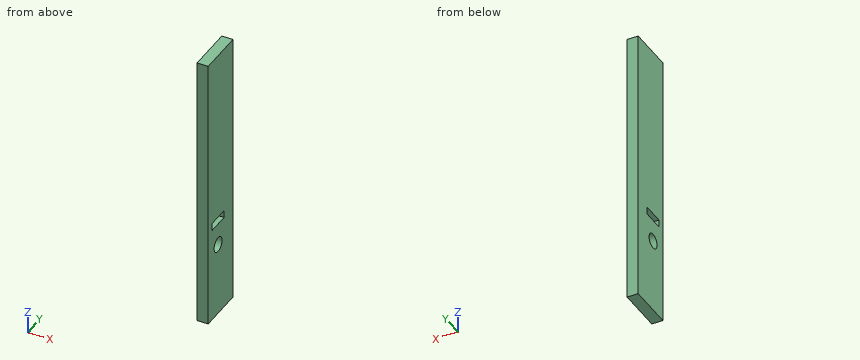
from build123d import *

# Parameters (mm, degrees)
SKETCH1_W           = 150
SKETCH1_H           = 25
SKETCH1_R           = 4
SKETCH1_W_2         = 4
SKETCH1_H_2         = 12
BOSS_EXTRUDE1_DEPTH = 6


with BuildPart() as part:
    # Sketch1 → Boss-Extrude1 (new body)
    with BuildSketch(Plane(origin=(0, 0, 0), x_dir=(0, 0, -1), z_dir=(1, 0, 0))):
        with Locations((75, 12.5)):
            Rectangle(SKETCH1_W, SKETCH1_H)
        with Locations((110, 10)):
            Circle(SKETCH1_R, mode=Mode.SUBTRACT)
        with Locations((96, 10)):
            Rectangle(SKETCH1_W_2, SKETCH1_H_2, mode=Mode.SUBTRACT)
    extrude(amount=BOSS_EXTRUDE1_DEPTH)


solid = part.part
The listing builds one solid part. Answer for the finished solid, in the listing's coordinates (mm). Coordinates: 2 decimals unless noted, no trailing zeros. Loops run counter-clockwise (first coordinate to the right, second up) from the corner with the lowest first, then second, coordinate; pieces in that order, holes last. Notation, with made-up numbers: M 48,50 L 102,50 A25 ccw 102,79 Z; hole C -9.75,-32 d5. An arc over 180 degrees is marked long. Answer in a Markdown table with one row per item.
1) Find section C-C (x = 2.4). Determine the outline of the cut face in (y, z), then the cut area to 3 significant figures.
Answers below:
| item | result |
|---|---|
| outline | M 0,-150 L 25,-150 L 25,0 L 0,0 Z; hole M 4,-98 L 16,-98 L 16,-94 L 4,-94 Z; hole C 10,-110 d8 |
| area | 3,650 mm^2 |
2) Find section A-A (y = 10). Determine the outline of the cut face in (x, z).
Answers below:
| item | result |
|---|---|
| outline | M 0,-150 L 6,-150 L 6,-114 L 0,-114 Z; M 0,-106 L 6,-106 L 6,-98 L 0,-98 Z; M 0,-94 L 6,-94 L 6,0 L 0,0 Z |
3) Find the intervals of material crossed by probe 1 along Y at (x, z) = (3.9, -110); probe 2 along Z at (x, y) = (1.55, 11); probe 3 along Y at (x, z) = (0.3, -97.5), in increasing order.
Answers below:
| item | result |
|---|---|
| probe 1 | 0 to 6, 14 to 25 |
| probe 2 | -150 to -113.87, -106.13 to -98, -94 to 0 |
| probe 3 | 0 to 4, 16 to 25 |
4) Find section B-B (z = -110). Determine the outline of the cut face in (x, y), then the cut area to 3 significant figures.
Answers below:
| item | result |
|---|---|
| outline | M 0,0 L 6,0 L 6,6 L 0,6 Z; M 0,14 L 6,14 L 6,25 L 0,25 Z |
| area | 102 mm^2 |
